Part model, mm, in its own coordinate system. A direction names the side the tool comes from. Coordinates: 2 decimals unless noted, no trailing zeros. Write each loop counter-clockwise with the first axis right and the second up, starting at its lowest first coordinate (ties: lowest second). Pieces come first, ordered by that corner, then holes. Notation, with made-up numbers: M 59.25,60 L 117.25,60 A17 ccw 117.25,72 Z; hole C -39,87.25 d1. An arc over 180 degrees is marked long. Use a Markdown table: item, result. Add a question column.
Q1. Slice it at B-B on y = -18.8. Write the cut outline in (x, z), then the cut area to 3 significant figures.
Q2. Pin check, flat tips, straight feed: pin 1 Ø3 at (x, y) = (42.78, -40.07) entering from -Z; pin 2 Ø1.5 at (x, z) = (-5, 1) entering from +Y. Stop position of each tip, or through.
Q3. Slice it at A-A on x = -1.5. Write the cut outline in (y, z).
Q4. Tool access for faces 1 (the flat face through (-4.514, -24, 2)), 2 (the flat face through (-29.71, 38.914, 1.521)), 3 (the flat face through (-40, 46.5, 1)): list every direction of +Z, -Z, +X, -X, +Y, -Y with a clear straight run to the whole face (end or side of a thin tool).
Q5. Wall check: L1, parallel to X at y = 37, z = 2.35; L2, parallel to Y at x = 17, z = 0.45; L3, parallel to X at y = -3.5, z = 2.6. Give the ranges that are in metal, low to high. Write a range as from..to.
Q6. Slice it at D-D on x = -33. Write the cut outline in (y, z).
Q7. Slice it at C-C on z = 1.05. Count the separate pieces of the cut face and the enclosed holes in it, then the cut area to 3 significant figures.
Q8. Mould opens along X. For faces 4 (the flat face through (-3.385, 24, 2)), 5 (the flat face through (-1, -10, 3)), 6 (the flat face through (-39.987, 0, 2)) say: released by +X, released by -X, zero draft, split by the parting line, or undercut.
from build123d import *

# Parameters (mm, degrees)
SKETCH1_W           = 92.97433
SKETCH1_H           = 93
BOSS_EXTRUDE1_DEPTH = 3
FILLET1_R           = 3
CUT_EXTRUDE1_DEPTH  = 3
SKETCH3_R           = 1.6
SKETCH3_R_2         = 1.65
SKETCH3_R_3         = 1.375
CUT_EXTRUDE2_DEPTH  = 3
SKETCH4_R           = 1.6
SKETCH4_R_2         = 1.65
SKETCH4_R_3         = 1.375
CUT_EXTRUDE3_DEPTH  = 3


with BuildPart() as part:
    # Sketch1 → Boss-Extrude1 (new body)
    with BuildSketch(Plane.XY):
        Rectangle(SKETCH1_W, SKETCH1_H)
    extrude(amount=BOSS_EXTRUDE1_DEPTH)

    # Fillet1
    fillet1_edges = [part.edges().sort_by_distance(p)[0] for p in [
        (46.487165, -46.5, 1.5),
        (-46.487165, -46.5, 1.5),
        (-46.487165, 46.5, 1.5),
        (46.487165, 46.5, 1.5),
    ]]
    fillet(fillet1_edges, radius=FILLET1_R)

    # Sketch2 → Cut-Extrude1 (cut)
    with BuildSketch(Plane.XY.offset(3)):
        Polygon((-39.987165, 30.80761), (-39.987165, -30.80761), (-9.179568981, 0), align=None)
        Polygon((-37.295165, 46.5), (-21.908517975, 31.113359908), (-7.648517975, 31.113359908), (-3.384663123, 26.849506978), (-3.384663123, 20.489506978), (-7.331622093, 16.54254623), (0.01788969, 9.193037759), (37.324835, 46.5), align=None)
        Polygon((30.474058677, -21.263117504), (39.987165, -7.74491836), (39.987165, 3.02508164), (35.150146737, 6.279640646), (35.150146737, 18.919640646), (31.628754168, 22.441031617), (9.199332158, 0.011599428), align=None)
        Polygon((-24.13996688, -33.24619021), (-30.87162192, -39.977848283), (30.93837808, -39.977358271), (0.122892986, -9.161887063), (-7.74013265, -17.024916241), (-4.514413398, -20.250634039), (-4.514413398, -27.320634039), (-10.43996688, -33.24619021), align=None)
    extrude(amount=-CUT_EXTRUDE1_DEPTH, mode=Mode.SUBTRACT)

    # Sketch3 → Cut-Extrude2 (cut)
    with BuildSketch(Plane.XY.offset(3)):
        with Locations((-42.887165, 37.38)):
            Circle(SKETCH3_R)
        with Locations((-32.877165, 32.89)):
            Circle(SKETCH3_R_2)
        with Locations((-19.987165, 24.3)):
            Circle(SKETCH3_R_3)
        with Locations((-10.187165, 24.3)):
            Circle(SKETCH3_R)
    extrude(amount=-CUT_EXTRUDE2_DEPTH, mode=Mode.SUBTRACT)

    # Sketch4 → Cut-Extrude3 (cut)
    with BuildSketch(Plane.XY.offset(3)):
        with Locations((42.777165, -40.07)):
            Circle(SKETCH4_R)
        with Locations((32.877165, -32.89)):
            Circle(SKETCH4_R_2)
        with Locations((37.987165, -24.5)):
            Circle(SKETCH4_R_3)
        with Locations((40.587165, -18.8)):
            Circle(SKETCH4_R)
        with Locations((-42.887165, -36.27)):
            Circle(SKETCH4_R)
        with Locations((-32.877165, -32.89)):
            Circle(SKETCH4_R_2)
        with Locations((-19.987165, -24.5)):
            Circle(SKETCH4_R_3)
        with Locations((-11.487165, -24)):
            Circle(SKETCH4_R)
        with Locations((42.777165, 39.9)):
            Circle(SKETCH4_R)
        with Locations((32.877165, 32.89)):
            Circle(SKETCH4_R_2)
        with Locations((37.987165, 24.5)):
            Circle(SKETCH4_R_3)
        with Locations((40.587165, 9.1)):
            Circle(SKETCH4_R)
    extrude(amount=-CUT_EXTRUDE3_DEPTH, mode=Mode.SUBTRACT)


solid = part.part
Recorded:
| question | item | result |
|---|---|---|
| 1 | outline | M -46.49,0 L -39.99,0 L -39.99,3 L -46.49,3 Z; M -27.98,0 L -5.97,0 L -5.97,3 L -27.98,3 Z; M 9.76,0 L 28.01,0 L 28.01,3 L 9.76,3 Z; M 32.21,0 L 38.99,0 L 38.99,3 L 32.21,3 Z; M 42.19,0 L 46.49,0 L 46.49,3 L 42.19,3 Z |
| 1 | area | 174 mm² |
| 2 | pin 1 | through |
| 2 | pin 2 | y = 29.21 |
| 3 | outline | M -46.5,0 L -39.98,0 L -39.98,3 L -46.5,3 Z; M -10.78,0 L 10.71,0 L 10.71,3 L -10.78,3 Z |
| 4 | face 1 | +Z, -Z |
| 4 | face 2 | +Z, -Z, +Y |
| 4 | face 3 | +Z, -Z, +X, -X, +Y |
| 5 | L1 | -46.49..-44.44, -41.33..-27.8, 27.82..46.49 |
| 5 | L2 | -46.5..-39.98, -26.04..-7.79, 7.81..26.18 |
| 5 | L3 | -46.49..-39.99, -12.68..12.71, 39.99..46.49 |
| 6 | outline | M -46.5,0 L -34.54,0 L -34.54,3 L -46.5,3 Z; M -31.24,0 L -23.82,0 L -23.82,3 L -31.24,3 Z; M 23.82,0 L 31.24,0 L 31.24,3 L 23.82,3 Z; M 34.54,0 L 42.2,0 L 42.2,3 L 34.54,3 Z |
| 7 | separate pieces | 1 |
| 7 | enclosed holes | 19 |
| 7 | area | 4,820 mm² |
| 8 | face 4 | undercut |
| 8 | face 5 | zero draft |
| 8 | face 6 | undercut |
